Model file for the job. Use its own axes, mm. A direction names the side the tool comes from. Round coordinates to 2 decimals unless told otherwise and drop trailing zeros. Order: outer loops, then holes, each group sorted by start corner. A loop starts at its lowest first (then second) coordinate and runs counter-clockwise, first axis right, second up. Notation, with made-up numbers: (-27, 63.5) - (25, 63.5) arc R18 ccw to (25, 71.5) - close; hole circle Ø8 at (-21, 70). An arc over 180 degrees is marked (long way). Write item = value, one per line.
```python
from build123d import *

# Parameters (mm, degrees)
SKETCH_R        = 24
SKETCH_R_2      = 4.5
SKETCH_R_3      = 2
PAD_DEPTH       = 11
CHAMFER_SIZE    = 2.1
FILLET_R        = 1.5
SKETCH001_R     = 8.5
POCKET_DEPTH    = 3
CHAMFER001_SIZE = 3.9


with BuildPart() as part:
    # Sketch → Pad (new body)
    with BuildSketch(Plane.XY):
        Circle(SKETCH_R)
        Circle(SKETCH_R_2, mode=Mode.SUBTRACT)
        with Locations((-12.15, 12.15)):
            Circle(SKETCH_R_3, mode=Mode.SUBTRACT)
        with Locations((12.15, 12.15)):
            Circle(SKETCH_R_3, mode=Mode.SUBTRACT)
        with Locations((12.15, -12.15)):
            Circle(SKETCH_R_3, mode=Mode.SUBTRACT)
        with Locations((-12.15, -12.15)):
            Circle(SKETCH_R_3, mode=Mode.SUBTRACT)
    extrude(amount=PAD_DEPTH)

    # Chamfer
    chamfer_edges = [part.edges().sort_by_distance(p)[0] for p in [
        (-14.15, 12.15, 11),
        (-14.15, -12.15, 11),
        (10.15, 12.15, 11),
        (10.15, -12.15, 11),
    ]]
    chamfer(chamfer_edges, length=CHAMFER_SIZE)

    # Fillet
    fillet_edges = [part.edges().sort_by_distance(p)[0] for p in [
        (-24, 0, 11),
    ]]
    fillet(fillet_edges, radius=FILLET_R)

    # Sketch001 (on Face10 of Fillet) → Pocket (cut)
    with BuildSketch(Plane(origin=(0, 0, 0), x_dir=(1, 0, 0), z_dir=(0, 0, -1))):
        Circle(SKETCH001_R)
    extrude(amount=-POCKET_DEPTH, mode=Mode.SUBTRACT)

    # Chamfer001
    chamfer001_edges = [part.edges().sort_by_distance(p)[0] for p in [
        (-4.5, 0, 3),
    ]]
    chamfer(chamfer001_edges, length=CHAMFER001_SIZE)


solid = part.part
```
1) Mould opens along X. For faces 3 (the face through (-13.624, -10.798, 4.388)), 4 (the face through (10, 0, 0)), 5 (the face through (-23.977, 1.055, 4.684)) say: +X half, -X half, draft (parallel to the pull), parting line (faces both ways), or undercut.
Conclusion:
face_3 = undercut
face_4 = draft
face_5 = parting line
2) Cut at B-B (x = -12.15). Give the number of separate pieces and of enclosed holes in the cut face, and give its area (3 significant figures).
Conclusion:
separate_pieces = 3
enclosed_holes = 0
area = 357 mm^2
3) 3-axis set-ups, long thin cutter, end or side, ignore diameter. For faces 1 (the face through (4.57, -7.167, 1.479)), 2 (the face through (13.225, -10.464, 4.388)): which of +Z, -Z, +X, -X, +Y, -Y reach the whole face in a straight line?
Conclusion:
face_1 = -Z
face_2 = +Z, -Z
4) Cut at A-A (z = 6). Write the cut outline in (x, y).
Conclusion:
outline = circle Ø48 at (0, 0); hole circle Ø4 at (-12.15, -12.15); hole circle Ø4 at (-12.15, 12.15); hole circle Ø10.8 at (0, 0); hole circle Ø4 at (12.15, -12.15); hole circle Ø4 at (12.15, 12.15)
5) Flat gauge pins, fed straight in: pin 1 Ø6 at (y, z) = (4.5, 7.5) entering from -X; pin 2 Ø4.5 at (x, y) = (12.15, -12.15) entering from -Z; pin 3 Ø1 at (x, z) = (-5, 6.5) entering from -Y; pin 4 Ø3 at (x, z) = (-7, 2) entering from +Y. Where does each tip first touch, or does it go through?
Conclusion:
pin_1 = -23.95
pin_2 = 0
pin_3 = -23.57
pin_4 = 23.36
6) Wall check: line 1 along Y through (x, z) = (0, 8.2); line 2 along Y through (x, z) = (12.15, 4.75); line 3 along Y through (x, z) = (-13, 10.75) (3 decimals). Give the ranges that are in metal, low to high.
Conclusion:
line_1 = -24 to -4.5, 4.5 to 24
line_2 = -20.7 to -14.15, -10.15 to 10.15, 14.15 to 20.7
line_3 = -19.371 to -15.905, -8.395 to 8.395, 15.905 to 19.371
